Here's how the part is built. I have some questions about the finished solid (model axes, mm). Face numbers are marked on the shaded views. A direction names the side the tool comes from. Coordinates: 2 decimals unless noted, no trailing zeros. Write each loop counter-clockwise with the first axis right and the second up, starting at its lowest first coordinate (ties: lowest second). Pieces come first, ordered by that corner, then holes. Notation, with made-up numbers: M 26.5,26.25 L 56.5,26.25 A19 ccw 56.5,48.25 Z; hole C 58,1 d5. An arc over 180 degrees is marked long. Use a Markdown table: item, result.
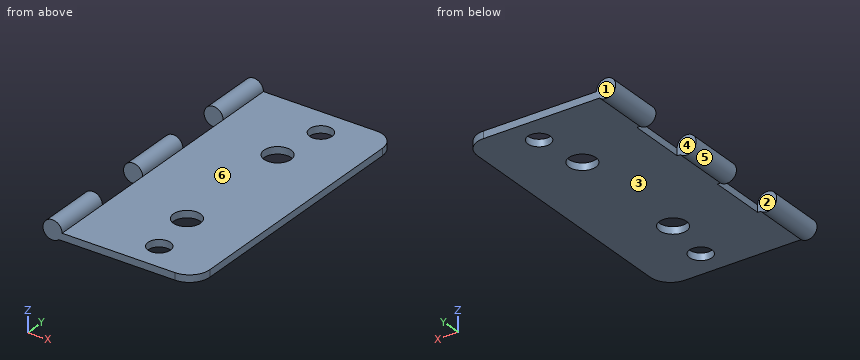
```python
from build123d import *

# Parameters (mm, degrees)
SKETCH1_R                = 2.97
SKETCH1_W                = 44.45
SKETCH1_H                = 2.2
BOSS_EXTRUDE1_DEPTH      = 44.45
CUT_EXTRUDE1_DEPTH       = 63.931914797
CUT_EXTRUDE1_DEPTH_BACK  = 63.931914797
SKETCH2_W                = 5.94
SKETCH2_H                = 17.78
FILLET1_R                = 6.35
SKETCH4_R                = 3.5
CUT_EXTRUDE2_DEPTH       = 63.931914797
F_5_16_CLEARANCE_HOLE1_D = 8.4328


with BuildPart() as part:
    # Sketch1 → Boss-Extrude1 (new, symmetric)
    with BuildSketch(Plane(origin=(0, 0, 0), x_dir=(1, 0, 0), z_dir=(0, 1, 0))):
        Circle(SKETCH1_R)
        with Locations((22.225, 1.1)):
            Rectangle(SKETCH1_W, SKETCH1_H)
    extrude(amount=BOSS_EXTRUDE1_DEPTH, both=True)

    # Sketch2 → Cut-Extrude1 (cut, two sides: drawn at the far end of the back side and taken through both)
    with BuildSketch(Plane.XY.offset(-CUT_EXTRUDE1_DEPTH_BACK)):
        with Locations((0, 17.78)):
            Rectangle(SKETCH2_W, SKETCH2_H)
        with Locations((0, -17.78)):
            Rectangle(SKETCH2_W, SKETCH2_H)
    extrude(amount=CUT_EXTRUDE1_DEPTH + CUT_EXTRUDE1_DEPTH_BACK, mode=Mode.SUBTRACT)

    # Fillet1
    fillet1_edges = [part.edges().sort_by_distance(p)[0] for p in [
        (44.45, 44.45, -1.1),
        (44.45, -44.45, -1.1),
    ]]
    fillet(fillet1_edges, radius=FILLET1_R)

    # Sketch4 → Cut-Extrude2 (cut, through all)
    with BuildSketch(Plane.XY):
        with Locations((27, 35.7)):
            Circle(SKETCH4_R)
        with Locations((27, -35.7)):
            Circle(SKETCH4_R)
    extrude(amount=-CUT_EXTRUDE2_DEPTH, mode=Mode.SUBTRACT)

    # 5/16 Clearance Hole1 (through all)
    with Locations(Plane.XY):
        with Locations((24.58125, 20.010345019), (24.58125, -20.010345019)):
            Hole(F_5_16_CLEARANCE_HOLE1_D / 2)


solid = part.part
```
1. Suppose I cut it at A-A on y = -35.7. Write out the boundary of the cut face in (x, z).
Answers follow:
| item | result |
|---|---|
| outline | M 2,-2.2 L 23.5,-2.2 L 23.5,0 L 2.97,0 A2.97 ccw long Z; M 30.5,-2.2 L 44.45,-2.2 L 44.45,0 L 30.5,0 Z |
2. I need wall thicknesses on probe 1 along Y at (x, z) = (22, -0.15); probe 2 along Z at (x, y) = (8, 37); probe 3 along X at (y, z) = (-34, 0.05). Which ranges of each line are inside material? Lowest first, please.
Answers follow:
| item | result |
|---|---|
| probe 1 | y = -44.45 to -23.34, -16.68 to 16.68, 23.34 to 44.45 |
| probe 2 | z = -2.2 to 0 |
| probe 3 | x = -2.97 to 2.97 |
3. Suppose I cut it at C-C on z = 2.1. Write out the boundary of the cut face in (x, y).
Answers follow:
| item | result |
|---|---|
| outline | M -2.1,-44.45 L 2.1,-44.45 L 2.1,-26.67 L -2.1,-26.67 Z; M -2.1,-8.89 L 2.1,-8.89 L 2.1,8.89 L -2.1,8.89 Z; M -2.1,26.67 L 2.1,26.67 L 2.1,44.45 L -2.1,44.45 Z |
4. We'd pull the mould along Y, two halves only. Please class the marked faces 1, 2 and 3: +Y half, -Y half, draft (parallel to the pull), parting line (faces both ways), or undercut.
Answers follow:
| item | result |
|---|---|
| face 1 | +Y half |
| face 2 | undercut |
| face 3 | draft |
5. Suppose I cut it at D-D on y = -7. Write out the boundary of the cut face in (x, z), and give its area (3 significant figures).
Answers follow:
| item | result |
|---|---|
| outline | M 2,-2.2 L 44.45,-2.2 L 44.45,0 L 2.97,0 A2.97 ccw long Z |
| area | 120 mm2 |
6. Will these pins go through, and if not, where does the flat tip stop? pin 1 Ø1.5 at (x, z) = (7, 0.5) entering from -Y; pin 2 Ø12 at (x, y) = (7.5, -31) entering from -Z; pin 3 Ø12.5 at (x, y) = (17.5, -1.5) entering from -Z; pin 4 Ø0.7 at (y, z) = (15.5, -1) entering from -X.
Answers follow:
| item | result |
|---|---|
| pin 1 | stops at y = -44.45 |
| pin 2 | stops at z = -2.56 |
| pin 3 | stops at z = -2.2 |
| pin 4 | stops at x = 2.97 |
7. Suppose I cut it at B-B on x = 26.5. Write out the boundary of the cut face in (y, z), and give its area (3 significant figures).
Answers follow:
| item | result |
|---|---|
| outline | M -44.45,-2.2 L -39.16,-2.2 L -39.16,0 L -44.45,0 Z; M -32.24,-2.2 L -23.76,-2.2 L -23.76,0 L -32.24,0 Z; M -16.26,-2.2 L 16.26,-2.2 L 16.26,0 L -16.26,0 Z; M 23.76,-2.2 L 32.24,-2.2 L 32.24,0 L 23.76,0 Z; M 39.16,-2.2 L 44.45,-2.2 L 44.45,0 L 39.16,0 Z |
| area | 132 mm2 |
8. Which directions (+Z, -Z, +X, -X, +Y, -Y) give clear straight access to the entire face, cutting with the end or side of a thin tool? Please do the marked faces 4, 5 and 6.
Answers follow:
| item | result |
|---|---|
| face 4 | +Z, -Z, -X |
| face 5 | +Y, -Y |
| face 6 | +Z, +X, +Y, -Y |
